For this review, take the finished solid that the model builds, in its own axes (mm). Round coordinates to 2 decimals unless told otherwise and drop trailing zeros. Write each loop counter-clockwise with the first axis right and the second up, starting at its lowest first coordinate (ties: lowest second). Pieces come first, ordered by that corner, then holes. Notation, with made-up numbers: (77, 28) -> (94, 28) arc R13 cw to (94, 48) -> close; hole circle Ø7 at (-28.5, 71.5). An arc over 180 degrees is marked (long way). Answer as CSV lines item,"result". Start each with the question number.
Item 1: Take a section at A-A on x = 0.35. Give the boundary of the cut face in (y, z).
Item 2: Wall thickness on probe 1 along Z at (x, y) = (0.2, -117.5); probe 2 along Y at (x, z) = (0.7, 95); probe 3 along Y at (x, z) = (0.8, -71.5) (3 decimals): over which ranges is each line inside the solid? List them lowest first. Write a range as from..to.
Item 3: Take a section at C-C on y = -151. Give the boundary of the cut face in (x, z), then the cut area to 3 significant figures.
Item 4: Take a section at B-B on z = 57. Give the boundary of the cut face in (x, y), then the cut area to 3 significant figures.
```python
from build123d import *

# Parameters (mm, degrees)
BOSS_EXTRUDE1_DEPTH   = 1
M4X0_7_TAPPED_HOLE1_D = 3.3


with BuildPart() as part:
    # Sketch1 → Boss-Extrude1 (new body)
    with BuildSketch(Plane(origin=(0, 0, 0), x_dir=(0, 0, -1), z_dir=(1, 0, 0))):
        Polygon((-100, 172.5), (-100, -172.5), (100, -122.5), (100, 172.5), align=None)
    extrude(amount=BOSS_EXTRUDE1_DEPTH)

    # M4x0.7 Tapped Hole1 (through all)
    with Locations(Plane(origin=(1, 0, 0), x_dir=(0, 0, -1), z_dir=(1, 0, 0))):
        with Locations((-95, 112.5), (-95, 102.5), (-95, -117.5), (-95, -127.5)):
            Hole(M4X0_7_TAPPED_HOLE1_D / 2)


solid = part.part
```
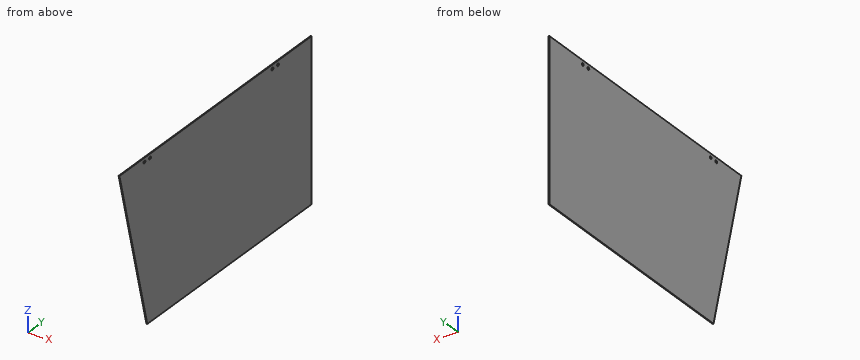
Output values:
1,outline,"(-172.5, 100) -> (-122.5, -100) -> (172.5, -100) -> (172.5, 100) -> close; hole circle Ø3.3 at (-127.5, 95); hole circle Ø3.3 at (-117.5, 95); hole circle Ø3.3 at (102.5, 95); hole circle Ø3.3 at (112.5, 95)"
2,probe 1,"z = -100..93.35, 96.65..100"
2,probe 2,"y = -171.25..-129.15, -125.85..-119.15, -115.85..100.85, 104.15..110.85, 114.15..172.5"
2,probe 3,"y = -129.625..172.5"
3,outline,"(0, 14) -> (1, 14) -> (1, 100) -> (0, 100) -> close"
3,area,"86.0 mm^2"
4,outline,"(0, -161.75) -> (1, -161.75) -> (1, 172.5) -> (0, 172.5) -> close"
4,area,"334 mm^2"
